The model under review builds one solid part; all positions refer to its coordinate system, in mm. Face numbers are marked on the shaded views. Round coordinates to 2 decimals unless told otherwise and drop trailing zeros. Order: outer loops, then holes, each group sorted by start corner. A loop starts at its lowest first (then second) coordinate and runs counter-clockwise, first axis right, second up. Notation, with made-up numbers: M 47,77.25 L 78,77.25 A22 cw 78,114.25 Z; hole C 74,7 d8. An arc over 180 degrees is marked long. Answer as a JSON object with one key per item and string values. Group by question number.
1) Consider section A-A, the plane x = 0. Write out the cut boundary in (y, z) (1 decimal).
2) The part is to be moulded in two halves that separate along Y. For the marked faces 1, 2 and 3, say which applies: +Y half, -Y half, draft (parallel to the pull), parting line (faces both ways), or undercut.
3) Consider section D-D, the plane y = 9.25. Write out the cut boundary in (x, z) (3 decimals).
4) Insertion check: pin 1 Ø1 at (y, z) = (11, 1.5) entering from -X; pin 2 Ø3 at (x, y) = (-5.5, 2) entering from -Z; pin 3 Ø4 at (x, y) = (-6.5, 5) entering from -Z (3 decimals). Each pin has a flat end and moves straight along its axis. Give the tip position at first contact, or say it passes through.
5) Consider section C-C, the plane x = 5.25. Write out the cut boundary in (y, z).
6) To check wall thickness, follow line 1 (Z direction, x = 0, y = 10) (3 decimals); line 2 (Y direction, x = 0, z = -8). State the ranges of each line that lie inside material, in increasing order.
7) Consider section B-B, the plane z = 0. Write out the cut boundary in (x, y) (3 decimals).
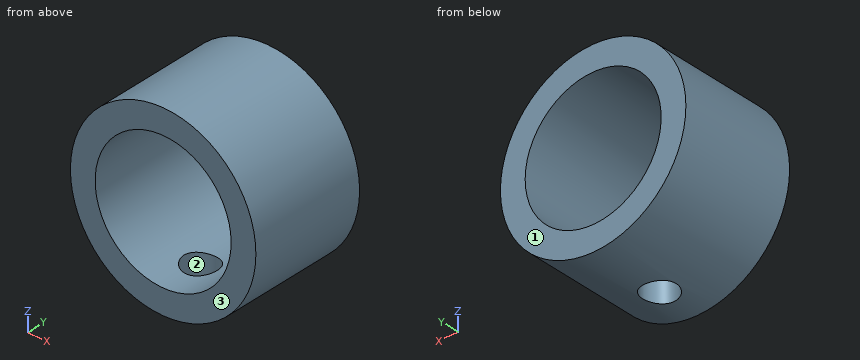
```python
from build123d import *

# Parameters (mm, degrees)
SKETCH1_R           = 9.525
SKETCH1_R_2         = 6.985
BOSS_EXTRUDE1_DEPTH = 4.445
SKETCH3_R           = 9.525
SKETCH3_R_2         = 6.985
BOSS_EXTRUDE2_DEPTH = 6.35
SKETCH2_R           = 1.7145
CUT_EXTRUDE1_DEPTH  = 10.525
SKETCH4_R           = 9.525
SKETCH4_R_2         = 6.985
BOSS_EXTRUDE3_DEPTH = 1.524


with BuildPart() as part:
    # Sketch1 → Boss-Extrude1 (new body)
    with BuildSketch(Plane(origin=(0, 0, 0), x_dir=(1, 0, 0), z_dir=(0, 1, 0))):
        Circle(SKETCH1_R)
        Circle(SKETCH1_R_2, mode=Mode.SUBTRACT)
    extrude(amount=BOSS_EXTRUDE1_DEPTH)

    # Sketch3 → Boss-Extrude2 (add)
    with BuildSketch(Plane(origin=(0, 4.445, 0), x_dir=(1, 0, 0), z_dir=(0, 1, 0))):
        Circle(SKETCH3_R)
        Circle(SKETCH3_R_2, mode=Mode.SUBTRACT)
    extrude(amount=BOSS_EXTRUDE2_DEPTH)

    # Sketch2 → Cut-Extrude1 (cut, through all)
    with BuildSketch(Plane.XY):
        with Locations((0, 4.445)):
            Circle(SKETCH2_R)
    extrude(amount=-CUT_EXTRUDE1_DEPTH, mode=Mode.SUBTRACT)

    # Sketch4 → Boss-Extrude3 (add)
    with BuildSketch(Plane(origin=(0, 10.795, 0), x_dir=(1, 0, 0), z_dir=(0, 1, 0))):
        Circle(SKETCH4_R)
        Circle(SKETCH4_R_2, mode=Mode.SUBTRACT)
    extrude(amount=BOSS_EXTRUDE3_DEPTH)


solid = part.part
```
Results list:
{
 "1": {"outline": "M 0,-9.5 L 2.7,-9.5 L 2.7,-7 L 0,-7 Z; M 0,7 L 12.3,7 L 12.3,9.5 L 0,9.5 Z; M 6.2,-9.5 L 12.3,-9.5 L 12.3,-7 L 6.2,-7 Z"},
 "2": {"face 1": "+Y half", "face 2": "undercut", "face 3": "-Y half"},
 "3": {"outline": "C 0,0 d19.05; hole C 0,0 d13.97"},
 "4": {"pin 1": "x = -9.47", "pin 2": "z = -8.64", "pin 3": "z = -8.395"},
 "5": {"outline": "M 0,-7.95 L 12.32,-7.95 L 12.32,-4.61 L 0,-4.61 Z; M 0,4.61 L 12.32,4.61 L 12.32,7.95 L 0,7.95 Z"},
 "6": {"line 1": "-9.525 to -6.985, 6.985 to 9.525", "line 2": "0 to 2.73, 6.16 to 12.32"},
 "7": {"outline": "M -9.525,0 L -6.985,0 L -6.985,12.319 L -9.525,12.319 Z; M 6.985,0 L 9.525,0 L 9.525,12.319 L 6.985,12.319 Z"}
}
